Autodesk Fusion 360 part; units mm, degrees
sketch "Sketch1" plane through (0, 0, 0) normal (0, 0, 1) x (1, 0, 0)
  circle A0 centre (0, 0) radius 4
  circle A1 centre (0, 0) radius 10
  line L0 (4, 0) -> (4, 9.1652)
  line L1 (-3.9998, -0.0353) -> (-4.0808, 9.1295)
  dimension "d1" = 8
  dimension "d2" = 20
extrude "Extrude1" add sketch "Sketch1" along normal blind 0.2 contours A0 A1 L0 L1 picked at (-7.9763, 0.257)
CAD build for the part. Positions are in the model's coordinates, mm. Round coordinates to 2 decimals unless told otherwise and drop trailing zeros. Order: outer loops, then holes, each group sorted by start corner. A loop starts at its lowest first (then second) coordinate and runs counter-clockwise, first axis right, second up. Notation, with made-up numbers: (65.25, 17.5) - (105.25, 17.5) arc R37 cw to (105.25, 55.5) - close; hole circle Ø8 at (63, 77.5). An arc over 180 degrees is marked (long way). Use CSV: the item, a comma, the result in double quotes. Start each with the question number.
1) Saw through at A-A (y = 1). List the corners of the cut face in (x, z).
2) Saw through at C-C (z = 0.1). List the corners of the cut face in (x, y), and give its area (3 significant figures).
3) Saw through at B-B (x = 0). List the corners of the cut face in (y, z), and give its area (3 significant figures).
4) Saw through at D-D (y = 3). List the corners of the cut face in (x, z), and give its area (3 significant figures).
5) Wall check: L1, parallel to X at y = -3, z = 0.1; L2, parallel to X at y = 3, z = 0.15; L3, parallel to Y at x = -1.75, z = 0.15. Give the ranges that are in metal, low to high. Write a range as [from, to].
Values follow:
1,outline,"(-9.95, 0) - (-4.01, 0) - (-4.01, 0.2) - (-9.95, 0.2) - close; (4, 0) - (9.95, 0) - (9.95, 0.2) - (4, 0.2) - close"
2,outline,"(-4.08, 9.13) arc R10 ccw (long way) to (4, 9.17) - (4, 0) arc R4 cw to (-4, -0.04) - close"
2,area,"211 mm2"
3,outline,"(-10, 0) - (-4, 0) - (-4, 0.2) - (-10, 0.2) - close"
3,area,"1.20 mm2"
4,outline,"(-9.54, 0) - (-4.03, 0) - (-4.03, 0.2) - (-9.54, 0.2) - close; (4, 0) - (9.54, 0) - (9.54, 0.2) - (4, 0.2) - close"
4,area,"2.21 mm2"
5,L1,"x = [-9.54, -2.65], [2.65, 9.54]"
5,L2,"x = [-9.54, -4.03], [4, 9.54]"
5,L3,"y = [-9.85, -3.6]"
